Verification items for the finished model (mm, model axes). A direction names the side the tool comes from. Coordinates: 2 decimals unless noted, no trailing zeros. Order: outer loops, then holes, each group sorted by start corner. A loop starts at its lowest first (then second) coordinate and runs counter-clockwise, first axis right, second up.
Q1. Cross-section at A-A, the plane x = 5. Record the boundary of the cut face in (y, z), and give its area (3 significant figures).
Q2. Set-up check for faces 1 (the flat face through (1, 5, -1)), 2 (the flat face through (6, 4.1, -22)), 3 (the flat face through (1, 15.2, -19)): record each of +Z, -Z, +X, -X, +Y, -Y from which the full face is reachable in a straight line by a thin tool's end or side.
Q3. Depth check by flat-ended pin: P1, Ø1.4, axis at y = 2.4, z = -17.8, coming from the -X side; P2, Ø0.6, axis at x = 1, y = 1, coming from the -Z side; P3, Ø1.6, axis at x = 0.5, y = 19, coming from the +Z side; P4, Ø6, axis at x = 30.5, y = 5, coming from the -Z side. Enter the tip coordinate at first touch or a pass-through.
Q4. Draft check along Y on faces 4 (the cylindrical face through (20.506, 18.593, -17.696)), 5 (the flat face through (19, 0, -10)), 6 (the flat face through (1, 1, -5)). Enter one of: pulls with the +Y half, pulls with the -Y half, needs draft (parallel to the pull), parting line crosses it, or undercut.
Q5. Cross-section at B-B, the plane z = -10.1. Record the boundary of the cut face in (x, y).
Q6. Cross-section at D-D, the plane z = -16.25. Record the boundary of the cut face in (x, y).
Q7. Cross-section at C-C, the plane y = 10.1. Record the boundary of the cut face in (x, z).
Q8. Thickness scan on line 1 (Z direction, x = 6, y = 2.5); line 2 (Y direction, x = 20, z = -17.8); line 3 (Y direction, x = 38.9, z = -10.1). Record the ranges inside material, lowest first.
from build123d import *

# Parameters (mm, degrees)
SKETCH_1_W          = 20.2
SKETCH_1_H          = 20.2
EXTRUDE_1_DEPTH     = 38.5
SKETCH_2_R          = 8
EXTRUDE_2_DEPTH     = 1.6
CUT_EXTRUDE_1_DEPTH = 2
M2X0_41_D           = 1.6
FILLET_1_R          = 2
SKETCH_7_R          = 2
CUT_EXTRUDE_2_DEPTH = 41.1
SKETCH_8_R          = 2.65
CUT_EXTRUDE_3_DEPTH = 5.5
SKETCH_9_R          = 3
CUT_EXTRUDE_4_DEPTH = 3
SKETCH_10_W         = 5
SKETCH_10_H         = 12
EXTRUDE_3_DEPTH     = 3.5


with BuildPart() as part:
    # Эскиз1 → Бобышка-Вытянуть1 (new body)
    with BuildSketch(Plane(origin=(0, 0, 0), x_dir=(0, 0, -1), z_dir=(1, 0, 0))):
        with Locations((10.1, 10.1)):
            Rectangle(SKETCH_1_W, SKETCH_1_H)
    extrude(amount=EXTRUDE_1_DEPTH)

    # Эскиз2 → Бобышка-Вытянуть2 (add)
    with BuildSketch(Plane(origin=(38.5, 0, 0), x_dir=(0, 0, -1), z_dir=(1, 0, 0))):
        with Locations((10.1, 10.1)):
            Circle(SKETCH_2_R)
    extrude(amount=EXTRUDE_2_DEPTH)

    # Эскиз3 → Вырез-Вытянуть1 (cut)
    with BuildSketch(Plane.ZY):
        with BuildLine():
            Line((-5, 20.2), (-5, 18.2))
            ThreePointArc((-5, 18.2), (-4.121320344, 16.078679656), (-2, 15.2))
            Line((-2, 15.2), (0, 15.2))
            Line((0, 15.2), (0, 20.2))
            Line((0, 20.2), (-5, 20.2))
        make_face()
        with BuildLine():
            Line((-20.2, 20.2), (-15.2, 20.2))
            Line((-15.2, 20.2), (-15.2, 18.2))
            ThreePointArc((-15.2, 18.2), (-16.078679656, 16.078679656), (-18.2, 15.2))
            Line((-18.2, 15.2), (-20.2, 15.2))
            Line((-20.2, 15.2), (-20.2, 20.2))
        make_face()
        with BuildLine():
            Line((0, 0), (-5, 0))
            Line((-5, 0), (-5, 2))
            ThreePointArc((-5, 2), (-4.121320344, 4.121320344), (-2, 5))
            Line((-2, 5), (0, 5))
            Line((0, 5), (0, 0))
        make_face()
        with BuildLine():
            Line((-15.2, 0), (-15.2, 2))
            ThreePointArc((-15.2, 2), (-16.078679656, 4.121320344), (-18.2, 5))
            Line((-18.2, 5), (-20.2, 5))
            Line((-20.2, 5), (-20.2, 0))
            Line((-20.2, 0), (-15.2, 0))
        make_face()
    extrude(amount=-CUT_EXTRUDE_1_DEPTH, mode=Mode.SUBTRACT)

    # Отверстие обработанное метчиком M2x0.41 (through all)
    with Locations(Plane.ZY.offset(-2)):
        with Locations((-17.8, 17.8), (-2.4, 17.8), (-2.4, 2.4), (-17.8, 2.4)):
            Hole(M2X0_41_D / 2)

    # Скругление1
    fillet_1_edges = [part.edges().sort_by_distance(p)[0] for p in [
        (20.25, 20.2, 0),
        (20.25, 20.2, -20.2),
        (20.25, 0, -20.2),
        (20.25, 0, 0),
    ]]
    fillet(fillet_1_edges, radius=FILLET_1_R)

    # Эскиз7 → Вырез-Вытянуть2 (cut, through all)
    with BuildSketch(Plane(origin=(40.1, 0, 0), x_dir=(0, 0, -1), z_dir=(1, 0, 0))):
        with Locations((10.1, 10.1)):
            Circle(SKETCH_7_R)
    extrude(amount=-CUT_EXTRUDE_2_DEPTH, mode=Mode.SUBTRACT)

    # Эскиз8 → Вырез-Вытянуть3 (cut)
    with BuildSketch(Plane.ZY):
        with Locations((-10.1, 10.1)):
            Circle(SKETCH_8_R)
    extrude(amount=-CUT_EXTRUDE_3_DEPTH, mode=Mode.SUBTRACT)

    # Эскиз9 → Вырез-Вытянуть4 (cut)
    with BuildSketch(Plane(origin=(40.1, 0, 0), x_dir=(0, 0, -1), z_dir=(1, 0, 0))):
        with Locations((10.1, 10.1)):
            Circle(SKETCH_9_R)
    extrude(amount=-CUT_EXTRUDE_4_DEPTH, mode=Mode.SUBTRACT)

    # Эскиз10 → Бобышка-Вытянуть3 (add)
    with BuildSketch(Plane(origin=(0, 0, -20.2), x_dir=(-1, 0, 0), z_dir=(0, 0, -1))):
        with Locations((-5.8, 10.1)):
            Rectangle(SKETCH_10_W, SKETCH_10_H)
    extrude(amount=EXTRUDE_3_DEPTH)


solid = part.part
Check values:
1. outline: (0, -18.2) arc R2 ccw to (2, -20.2) - (4.1, -20.2) - (4.1, -23.7) - (16.1, -23.7) - (16.1, -20.2) - (18.2, -20.2) arc R2 ccw to (20.2, -18.2) - (20.2, -2) arc R2 ccw to (18.2, 0) - (2, 0) arc R2 ccw to (0, -2) - close; hole circle Ø1.6 at (2.4, -17.8); hole circle Ø1.6 at (2.4, -2.4); hole circle Ø5.3 at (10.1, -10.1); hole circle Ø1.6 at (17.8, -17.8); hole circle Ø1.6 at (17.8, -2.4)
1. area: 417 mm2
2. face 1: +Z, -X, -Y
2. face 2: -Z, +X, -X, -Y
2. face 3: -Z, -X, +Y
3. P1: passes through
3. P2: stops at z = -15.2
3. P3: stops at z = -5
3. P4: stops at z = -20.2
4. face 4: undercut
4. face 5: pulls with the -Y half
4. face 6: needs draft
5. outline: (0, 0) - (38.5, 0) - (38.5, 2.1) - (40.1, 2.1) - (40.1, 7.1) - (37.1, 7.1) - (37.1, 8.1) - (5.5, 8.1) - (5.5, 7.45) - (0, 7.45) - close; (0, 12.75) - (5.5, 12.75) - (5.5, 12.1) - (37.1, 12.1) - (37.1, 13.1) - (40.1, 13.1) - (40.1, 18.1) - (38.5, 18.1) - (38.5, 20.2) - (0, 20.2) - close
6. outline: (0, 4.28) - (2, 4.28) - (2, 0) - (38.5, 0) - (38.5, 4.98) - (40.1, 4.98) - (40.1, 15.22) - (38.5, 15.22) - (38.5, 20.2) - (2, 20.2) - (2, 15.92) - (0, 15.92) - close
7. outline: (0, -20.2) - (3.3, -20.2) - (3.3, -23.7) - (8.3, -23.7) - (8.3, -20.2) - (38.5, -20.2) - (38.5, -18.1) - (40.1, -18.1) - (40.1, -13.1) - (37.1, -13.1) - (37.1, -12.1) - (5.5, -12.1) - (5.5, -12.75) - (0, -12.75) - close; (0, -7.45) - (5.5, -7.45) - (5.5, -8.1) - (37.1, -8.1) - (37.1, -7.1) - (40.1, -7.1) - (40.1, -2.1) - (38.5, -2.1) - (38.5, 0) - (0, 0) - close
8. line 1: z = -20.2 to -18.59, -17.01 to -3.19, -1.61 to 0
8. line 2: y = 0 to 1.6, 3.2 to 17, 18.6 to 20.2
8. line 3: y = 2.1 to 7.1, 13.1 to 18.1
